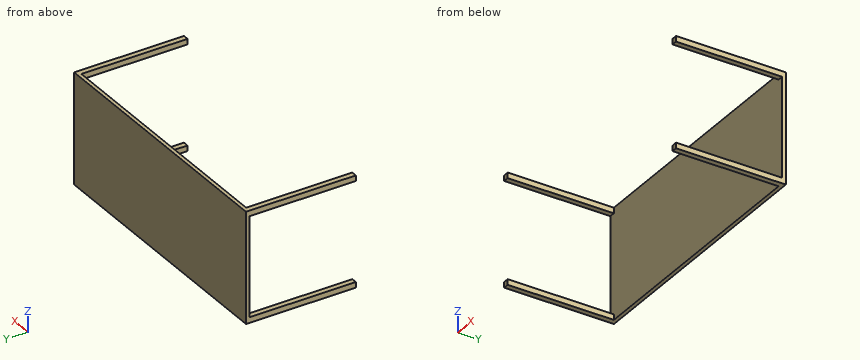
```python
from build123d import *

# Parameters (mm, degrees)
SKETCH1_W           = 1854.2
SKETCH1_H           = 762
BOSS_EXTRUDE1_DEPTH = 756.92
CUT_EXTRUDE1_DEPTH  = 731.52


with BuildPart() as part:
    # Sketch1 → Boss-Extrude1 (new body)
    with BuildSketch(Plane(origin=(0, 0, 0), x_dir=(1, 0, 0), z_dir=(0, 1, 0))):
        Rectangle(SKETCH1_W, SKETCH1_H)
    extrude(amount=BOSS_EXTRUDE1_DEPTH)

    # Sketch2 → Cut-Extrude1 (cut)
    with BuildSketch(Plane.XZ):
        Polygon((-889, 381), (889, 381), (889, 342.9), (927.1, 342.9), (927.1, -342.9), (889, -342.9), (889, -381), (-889, -381), (-889, -342.9), (-927.1, -342.9), (-927.1, 342.9), (-889, 342.9), align=None)
    extrude(amount=-CUT_EXTRUDE1_DEPTH, mode=Mode.SUBTRACT)


solid = part.part
```
The listing builds one solid part. Answer for the finished solid, in the listing's coordinates (mm). Round coordinates to 2 decimals unless told otherwise and drop trailing zeros. Loops run counter-clockwise (first coordinate to the right, second up) from the corner with the lowest first, then second, coordinate; pieces in that order, holes last.
1) Given P1, Ø12, axis at x = -661.5, z = -161.5, coming from the -Y side, flat-ended and moving along its own axis, determine where the tip first touches the part or whether it passes through.
Outcome:
P1: stops at y = 731.52
2) A cutting plane is placed at C-C on z = -3.5. Determine the outline of the cut face in (x, y).
Outcome:
outline: (-927.1, 731.52) - (927.1, 731.52) - (927.1, 756.92) - (-927.1, 756.92) - close
3) A cutting plane is placed at A-A on y = 358.5. Determine the outline of the cut face in (x, z), plus the area to 3 significant figures.
Outcome:
outline: (-927.1, -381) - (-889, -381) - (-889, -342.9) - (-927.1, -342.9) - close; (-927.1, 342.9) - (-889, 342.9) - (-889, 381) - (-927.1, 381) - close; (889, -381) - (927.1, -381) - (927.1, -342.9) - (889, -342.9) - close; (889, 342.9) - (927.1, 342.9) - (927.1, 381) - (889, 381) - close
area: 5,810 mm2
4) A cutting plane is placed at B-B on x = 132. Determine the outline of the cut face in (y, z), plus the area to 3 significant figures.
Outcome:
outline: (731.52, -381) - (756.92, -381) - (756.92, 381) - (731.52, 381) - close
area: 19,400 mm2
5) Consider line 1 (Y direction, x = 830, z = -94.5). Determine where the line is inside the solid, lowest interval first.
Outcome:
line 1: y = 731.52 to 756.92
